```python
from build123d import *

# Parameters (mm, degrees)
BOX101_W     = 3
BOX101_H     = 4
BOX101_DEPTH = 6
BOX060_W     = 3
BOX060_H     = 6
BOX060_DEPTH = 5
BOX061_W     = 3
BOX061_H     = 6
BOX061_DEPTH = 5
BOX063_W     = 3
BOX063_H     = 6
BOX063_DEPTH = 5
BOX062_W     = 3
BOX062_H     = 6
BOX062_DEPTH = 5
BOX058_W     = 3
BOX058_H     = 6
BOX058_DEPTH = 5
BOX059_W     = 3
BOX059_H     = 6
BOX059_DEPTH = 5
BOX056_W     = 3
BOX056_H     = 6
BOX056_DEPTH = 5
BOX026_W     = 5
BOX026_H     = 7
BOX026_DEPTH = 7
BOX020_W     = 6
BOX020_H     = 4
BOX020_DEPTH = 6
BOX_W        = 43
BOX_H        = 23
BOX_DEPTH    = 10
BOX001_W     = 45
BOX001_H     = 25
BOX001_DEPTH = 10


with BuildPart() as box101:
    # Box101 → Box101 (new body)
    with BuildSketch(Plane(origin=(0, 3, 2), x_dir=(1, 0, 0), z_dir=(0, 0, 1))):
        with Locations((1.5, 2)):
            Rectangle(BOX101_W, BOX101_H)
    extrude(amount=BOX101_DEPTH)


with BuildPart() as box060:
    # Box060 → Box060 (new body)
    with BuildSketch(Plane(origin=(29, -2, 3), x_dir=(1, 0, 0), z_dir=(0, 0, 1))):
        with Locations((1.5, 3)):
            Rectangle(BOX060_W, BOX060_H)
    extrude(amount=BOX060_DEPTH)


with BuildPart() as box061:
    # Box061 → Box061 (new body)
    with BuildSketch(Plane(origin=(38, -2, 3), x_dir=(1, 0, 0), z_dir=(0, 0, 1))):
        with Locations((1.5, 3)):
            Rectangle(BOX061_W, BOX061_H)
    extrude(amount=BOX061_DEPTH)


with BuildPart() as box063:
    # Box063 → Box063 (new body)
    with BuildSketch(Plane(origin=(46, 11, 3), x_dir=(0, 1, 0), z_dir=(0, 0, 1))):
        with Locations((1.5, 3)):
            Rectangle(BOX063_W, BOX063_H)
    extrude(amount=BOX063_DEPTH)


with BuildPart() as box062:
    # Box062 → Box062 (new body)
    with BuildSketch(Plane(origin=(46, 4, 3), x_dir=(0, 1, 0), z_dir=(0, 0, 1))):
        with Locations((1.5, 3)):
            Rectangle(BOX062_W, BOX062_H)
    extrude(amount=BOX062_DEPTH)


with BuildPart() as box058:
    # Box058 → Box058 (new body)
    with BuildSketch(Plane(origin=(12, -2, 3), x_dir=(1, 0, 0), z_dir=(0, 0, 1))):
        with Locations((1.5, 3)):
            Rectangle(BOX058_W, BOX058_H)
    extrude(amount=BOX058_DEPTH)


with BuildPart() as box059:
    # Box059 → Box059 (new body)
    with BuildSketch(Plane(origin=(20, -2, 3), x_dir=(1, 0, 0), z_dir=(0, 0, 1))):
        with Locations((1.5, 3)):
            Rectangle(BOX059_W, BOX059_H)
    extrude(amount=BOX059_DEPTH)


with BuildPart() as box056:
    # Box056 → Box056 (new body)
    with BuildSketch(Plane(origin=(16, 20, 3), x_dir=(1, 0, 0), z_dir=(0, 0, 1))):
        with Locations((1.5, 3)):
            Rectangle(BOX056_W, BOX056_H)
    extrude(amount=BOX056_DEPTH)


with BuildPart() as box026:
    # Box026 → Box026 (new body)
    with BuildSketch(Plane(origin=(4, 20, 1), x_dir=(1, 0, 0), z_dir=(0, 0, 1))):
        with Locations((2.5, 3.5)):
            Rectangle(BOX026_W, BOX026_H)
    extrude(amount=BOX026_DEPTH)


with BuildPart() as box020:
    # Box020 → Box020 (new body)
    with BuildSketch(Plane(origin=(-2, 10, 2), x_dir=(1, 0, 0), z_dir=(0, 0, 1))):
        with Locations((3, 2)):
            Rectangle(BOX020_W, BOX020_H)
    extrude(amount=BOX020_DEPTH)


with BuildPart() as box:
    # Box → Box (new body)
    with BuildSketch(Plane(origin=(1, 1, 1), x_dir=(1, 0, 0), z_dir=(0, 0, 1))):
        with Locations((21.5, 11.5)):
            Rectangle(BOX_W, BOX_H)
    extrude(amount=BOX_DEPTH)


with BuildPart() as cut037:
    # Box001 → Box001 (new body)
    with BuildSketch(Plane.XY):
        with Locations((22.5, 12.5)):
            Rectangle(BOX001_W, BOX001_H)
    extrude(amount=BOX001_DEPTH)

    # Cut: cut Box
    add(box.part, mode=Mode.SUBTRACT)

    # Cut001: cut Box020
    add(box020.part, mode=Mode.SUBTRACT)

    # Cut029: cut Box026
    add(box026.part, mode=Mode.SUBTRACT)

    # Cut030: cut Box056
    add(box056.part, mode=Mode.SUBTRACT)

    # Cut031: cut Box059
    add(box059.part, mode=Mode.SUBTRACT)

    # Cut032: cut Box058
    add(box058.part, mode=Mode.SUBTRACT)

    # Cut033: cut Box062
    add(box062.part, mode=Mode.SUBTRACT)

    # Cut034: cut Box063
    add(box063.part, mode=Mode.SUBTRACT)

    # Cut035: cut Box061
    add(box061.part, mode=Mode.SUBTRACT)

    # Cut036: cut Box060
    add(box060.part, mode=Mode.SUBTRACT)

    # Cut037: cut Box101
    add(box101.part, mode=Mode.SUBTRACT)


solid = cut037.part
```
Geometry check sheet. Reference: the model listing, model coordinates, mm. A direction names the side the tool comes from. Coordinates: 2 decimals unless noted, no trailing zeros. Order: outer loops, then holes, each group sorted by start corner. A loop starts at its lowest first (then second) coordinate and runs counter-clockwise, first axis right, second up. Notation, with made-up numbers: (13, 89.5) - (24, 89.5) arc R35 ccw to (24, 124.5) - close; hole circle Ø2 at (37, 33). An arc over 180 degrees is marked (long way). Answer as a JSON object with one key per item and string values. Group by question number.
Item 1: Sectioned sample at D-D, the plane z = 6. Give the number of separate pieces and of enclosed holes in the cut face, and give its area (3 significant figures).
Item 2: Scan lines: probe 1 along X at (y, z) = (18, 6.5); probe 2 along Y at (x, z) = (19, 2.5); probe 3 along Z at (x, y) = (13.5, 18). Record each from-to range of solid material in increasing order.
Item 3: Sectioned sample at B-B, the plane y = 6. Record the cut outline in (x, z), and give its area (3 significant figures).
Item 4: Draft check along X on faces 5 (the face through (39.5, 0.5, 3)), 6 (the face through (0.5, 14, 5)), 7 (the face through (17.5, 24.5, 8)), 8 (the face through (0, 15, 5)). Enter one of: +X half, -X half, draft (parallel to the pull), parting line (faces both ways), or undercut.
Item 5: Sectioned sample at C-C, the plane y = 20.5. Record the cut outline in (x, z), and give its area (3 significant figures).
Item 6: Tool access check on faces 1 (the face through (0.5, 12, 2)), 2 (the face through (44.5, 5.5, 8)), 3 (the face through (4, 24.5, 4.5)), 4 (the face through (29, 0.5, 5.5)). Record the directions out of +Z, -Z, +X, -X, +Y, -Y that give a thin tool (end or side, any length) a straight path to the whole face; none if there is none.
Item 7: Depth check by flat-ended pin: pin 1 Ø5 at (x, y) = (21, 9) entering from +Z. Enter the tip coordinate at first touch or a pass-through.
Item 8: Sectioned sample at A-A, the plane x = 8.5. Record the cut outline in (y, z).
Resolved:
{
 "1": {"separate pieces": "10", "enclosed holes": "0", "area": "102 mm^2"},
 "2": {"probe 1": "0 to 1, 44 to 45", "probe 2": "0 to 1, 24 to 25", "probe 3": "0 to 1"},
 "3": {"outline": "(0, 0) - (45, 0) - (45, 3) - (44, 3) - (44, 1) - (1, 1) - (1, 2) - (0, 2) - close; (0, 8) - (1, 8) - (1, 10) - (0, 10) - close; (44, 8) - (45, 8) - (45, 10) - (44, 10) - close", "area": "52.0 mm^2"},
 "4": {"face 5": "undercut", "face 6": "draft", "face 7": "undercut", "face 8": "-X half"},
 "5": {"outline": "(0, 0) - (45, 0) - (45, 10) - (44, 10) - (44, 1) - (1, 1) - (1, 10) - (0, 10) - close", "area": "63.0 mm^2"},
 "6": {"face 1": "-X", "face 2": "+X, -X", "face 3": "+Y", "face 4": "-Y"},
 "7": {"pin 1": "z = 1"},
 "8": {"outline": "(0, 0) - (25, 0) - (25, 1) - (1, 1) - (1, 10) - (0, 10) - close; (24, 8) - (25, 8) - (25, 10) - (24, 10) - close"}
}
